from build123d import *

# Parameters (mm, degrees)
BOSS_EXTRUDE1_DEPTH   = 12.7
F_8_CLEARANCE_HOLE1_D = 4.9149
F_8_CLEARANCE_HOLE2_D = 4.9149


with BuildPart() as part:
    # Sketch1 → Boss-Extrude1 (new body)
    with BuildSketch(Plane.XY):
        Polygon((-3.452609544, 16.036650639), (-3.452609544, -3.013349361), (15.597390456, -3.013349361), (15.597390456, -1.413149361), (-1.852409544, -1.413149361), (-1.852409544, 16.036650639), align=None)
    extrude(amount=BOSS_EXTRUDE1_DEPTH)

    # #8 Clearance Hole1 (through all)
    with Locations(Plane(origin=(0, -1.413149361, 0), x_dir=(1, 0, 0), z_dir=(0, 1, 0))):
        with Locations((6.072390456, -6.35)):
            Hole(F_8_CLEARANCE_HOLE1_D / 2)

    # #8 Clearance Hole2 (through all)
    with Locations(Plane(origin=(-1.852409544, 0, 0), x_dir=(0, 0, -1), z_dir=(1, 0, 0))):
        with Locations((-6.35, 6.384650639)):
            Hole(F_8_CLEARANCE_HOLE2_D / 2)


solid = part.part
Here's how the part is built. I have some questions about the finished solid (model axes, mm). A direction names the side the tool comes from. Round coordinates to 2 decimals unless told otherwise and drop trailing zeros. Loops run counter-clockwise (first coordinate to the right, second up) from the corner with the lowest first, then second, coordinate; pieces in that order, holes last.
1. If we section it at B-B on x = 4: Write out the boundary of the cut face in (y, z).
Answer list:
outline: (-3.01, 0) - (-1.41, 0) - (-1.41, 5.03) - (-3.01, 5.03) - close; (-3.01, 7.67) - (-1.41, 7.67) - (-1.41, 12.7) - (-3.01, 12.7) - close
2. If I drill on line 1 along Y through (x, z) = (-2.75, 6.35); line 2 along Y through (x, z) = (1, 8.5); line 3 along X through (y, z) = (8.75, 2), over which ranges is the centre line in solid material (lowest first)?
Answer list:
line 1: y = -3.01 to 3.93, 8.84 to 16.04
line 2: y = -3.01 to -1.41
line 3: x = -3.45 to -1.85
3. If we section it at A-A on z = 6.35: Write out the boundary of the cut face in (x, y), plus the area to 3 significant figures.
Answer list:
outline: (-3.45, -3.01) - (3.61, -3.01) - (3.61, -1.41) - (-1.85, -1.41) - (-1.85, 3.93) - (-3.45, 3.93) - close; (-3.45, 8.84) - (-1.85, 8.84) - (-1.85, 16.04) - (-3.45, 16.04) - close; (8.53, -3.01) - (15.6, -3.01) - (15.6, -1.41) - (8.53, -1.41) - close
area: 42.7 mm2
4. We'd pull the mould along Z, two halves only. Please class faces 1 (the face through (-2.4, 2.3, 12.7)), 2 (the face through (4.75, -2.22, 4.28)), 3 (the face through (-2.66, 8.82, 6.03)), 4 (the face through (-3, 16.037, 6)): +Z half, -Z half, draft (parallel to the pull), parting line (faces both ways), or undercut.
Answer list:
face 1: +Z half
face 2: undercut
face 3: undercut
face 4: draft
5. For P1, Ø4, axis at y = 10, z = 9, coming from the +X side; P2, Ø6.5, axis at x = 5, z = 4, coming from the +Y side, each with a flat end and sliding along its axis, tell me the tip position at first contact or that it passes through.
Answer list:
P1: stops at x = -1.85
P2: stops at y = -1.41
6. If we section it at D-D on y = 1.5: Write out the boundary of the cut face in (x, z), plus the area to 3 significant figures.
Answer list:
outline: (-3.45, 0) - (-1.85, 0) - (-1.85, 12.7) - (-3.45, 12.7) - close
area: 20.3 mm2
7. Which directions (+Z, -Z, +X, -X, +Y, -Y) give clear straight access to the entire face, cutting with the end or side of a thin tool? Please do faces 5 (the face through (-2.4, 2.3, 0)), 6 (the face through (-1.852, 9, 6)).
Answer list:
face 5: -Z, +X, -X, +Y, -Y
face 6: +Z, -Z, +X, +Y
8. If we section it at C-C on z = 11.75: Write out the boundary of the cut face in (x, y), plus the area to 3 significant figures.
Answer list:
outline: (-3.45, -3.01) - (15.6, -3.01) - (15.6, -1.41) - (-1.85, -1.41) - (-1.85, 16.04) - (-3.45, 16.04) - close
area: 58.4 mm2
